CAD build for the part. Positions are in the model's coordinates, mm. A direction names the side the tool comes from. Round coordinates to 2 decimals unless told otherwise and drop trailing zeros. Order: outer loops, then holes, each group sorted by start corner. A loop starts at its lowest first (then second) coordinate and runs counter-clockwise, first axis right, second up. Notation, with made-up numbers: M -1,-13 L 37,-13 A22 ccw 37,-5 Z; hole C 51,86 d7. An arc over 180 degrees is marked long. Answer as a JSON object with one key per item and string values.
```python
from build123d import *

# Parameters (mm, degrees)
EXTRUDE_1_DEPTH     = 5
FILLET_1_R          = 2.5
EXTRUDE_2_DEPTH     = 8
FILLET_3_R          = 2.5
SKETCH_5_W          = 1.467751534
SKETCH_5_H          = 4.178210798
SKETCH_5_W_2        = 1.389566385
CUT_EXTRUDE_1_DEPTH = 20
EXTRUDE_3_DEPTH     = 38
SKETCH_7_W          = 2.4
SKETCH_7_H          = 1.7
CUT_EXTRUDE_2_DEPTH = 38


with BuildPart() as part:
    # 草图1 → 凸台-拉伸1 (new body)
    with BuildSketch(Plane.XY):
        Polygon((0, 0), (0, 28), (4, 28), (7.380946094, 20.749537704), (11.912485029, 22.862629012), (7.185351304, 33), (-5, 33), (-5, -5), (8, -5), (8, 0), align=None)
    extrude(amount=EXTRUDE_1_DEPTH)

    # 圆角1
    fillet_1_edges = [part.edges().sort_by_distance(p)[0] for p in [
        (9.646715562, 21.806083358, 0),
        (7.185351304, 33, 2.5),
        (11.912485029, 22.862629012, 2.5),
        (7.380946094, 20.749537704, 2.5),
        (9.646715562, 21.806083358, 5),
    ]]
    fillet(fillet_1_edges, radius=FILLET_1_R - 0.0001)  # a hair under: the kernel refuses the full size

    # 草图3 → 凸台-拉伸2 (add)
    with BuildSketch(Plane(origin=(0, 0, 0), x_dir=(0, 0, -1), z_dir=(1, 0, 0))):
        with BuildLine():
            Line((-5, 0), (0, 0))
            ThreePointArc((0, 0), (-2.5, 2.5), (-5, 0))
        make_face()
    extrude(amount=EXTRUDE_2_DEPTH)

    # 圆角3
    fillet_3_edges = [part.edges().sort_by_distance(p)[0] for p in [
        (8, -2.5, 0),
        (8, -5, 2.5),
        (8, -2.5, 5),
        (8, 2.5, 2.5),
    ]]
    fillet(fillet_3_edges, radius=FILLET_3_R - 0.0001)  # a hair under: the kernel refuses the full size

    # 草图4 → 旋转3 (revolve)
    with BuildSketch(Plane(origin=(4.4, 0, 0), x_dir=(0, 0, -1), z_dir=(1, 0, 0))):
        with BuildLine():
            Line((-5.5, 0), (0.5, 0))
            ThreePointArc((0.5, 0), (-2.5, 3), (-5.5, 0))
        make_face()
    revolve(axis=Axis((4.4, 0, 2.5), (0, 0, -1)))

    # 草图5 → 切除-拉伸1 (cut)
    with BuildSketch(Plane.ZY.offset(5)):
        with Locations((-0.733875767, -0.010051234)):
            Rectangle(SKETCH_5_W, SKETCH_5_H)
        with Locations((5.694783193, -0.010051234)):
            Rectangle(SKETCH_5_W_2, SKETCH_5_H)
    extrude(amount=-CUT_EXTRUDE_1_DEPTH, mode=Mode.SUBTRACT)

    # 草图6 → 凸台-拉伸3 (add)
    with BuildSketch(Plane.XZ.offset(5)):
        Polygon((-5, 2.5), (-5, 3.5), (-7, 3.5), (-7, 5), (-9, 5), (-11.5, 2.5), (-9, 0), (-7, 0), (-7, 1.5), (-5, 1.5), align=None)
    extrude(amount=-EXTRUDE_3_DEPTH)

    # 草图7 → 切除-拉伸2 (cut)
    with BuildSketch(Plane.XZ.offset(5)):
        with Locations((-6, 4.15)):
            Rectangle(SKETCH_7_W, SKETCH_7_H)
        with Locations((-6, 0.85)):
            Rectangle(SKETCH_7_W, SKETCH_7_H)
    extrude(amount=-CUT_EXTRUDE_2_DEPTH, mode=Mode.SUBTRACT)


solid = part.part
```
Item 1: Drop flat-ended pins along their axis: pin 1 Ø1.9 at (y, z) = (9.5, 4) entering from -X; pin 2 Ø0.8 at (y, z) = (5.5, 4.5) entering from +X; pin 3 Ø1.4 at (y, z) = (9, 0.5) entering from -X. Give the stop position or say it passes through.
Worked answers:
{"pin 1": "stops at x = -10.95", "pin 2": "stops at x = 0", "pin 3": "stops at x = -10.2"}
Item 2: 3-axis set-ups, long thin cutter, end or side, ignore diameter. For faces 1 (the flat face through (5.146, 25.543, 2.465)), 2 (the flat face through (-7.2, 14, 4)), 3 (the cylindrical face through (7.248, -1.979, 4.287)): which of +Z, -Z, +X, -X, +Y, -Y reach the whole face in a straight line?
Worked answers:
{"face 1": "+Z, -Z", "face 2": "+Z, +Y, -Y", "face 3": "+Z, +X, -Y"}
Item 3: Saw through at B-B on y = 27.5. List the corners of the cut face in (x, z).
Worked answers:
{"outline": "M -11.5,2.5 L -9,0 L -7.2,0 L -7.2,1.7 L -4.8,1.7 L -4.8,0 L 0,0 L 0,5 L -4.8,5 L -4.8,3.3 L -7.2,3.3 L -7.2,5 L -9,5 Z; M 4.23,0 L 9.75,0 L 9.75,5 L 4.23,5 Z"}
Item 4: Wall check: line 1 along X through (y, z) = (26.5, 0.7); line 2 along X through (y, z) = (23, 4.05); line 3 along Y through (x, z) = (1, 2.55). Give the ranges that are in metal, low to high. Write a range as [from, to].
Worked answers:
{"line 1": "x = [-9.7, -7.2], [-4.8, 0], [4.7, 10.22]", "line 2": "x = [-9.95, -7.2], [-4.8, 0], [6.33, 10.85]", "line 3": "y = [-5, 2.5], [28, 33]"}
Item 5: Saw through at C-C on y = 12. List the corners of the cut face in (x, z).
Worked answers:
{"outline": "M -11.5,2.5 L -9,0 L -7.2,0 L -7.2,1.7 L -4.8,1.7 L -4.8,0 L 0,0 L 0,5 L -4.8,5 L -4.8,3.3 L -7.2,3.3 L -7.2,5 L -9,5 Z"}
Item 6: Saw through at D-D on x = -5.5. List the corners of the cut face in (y, z), and give its area (3 significant figures).
Worked answers:
{"outline": "M -5,1.7 L 33,1.7 L 33,3.3 L -5,3.3 Z", "area": "60.8 mm2"}
Item 7: Two-plate mould, pull along Y, no slides. Class faces 4 (the cylindrical face through (1.4, 2.5, 2.4)), 5 (the flat face through (-1, 14, 5)), 6 (the flat face through (-1, 33, 2)), 7 (the cylindrical face through (9.237, 22.767, 4.532)): released by +Y, released by -Y, zero draft, split by the parting line, or undercut.
Worked answers:
{"face 4": "undercut", "face 5": "zero draft", "face 6": "released by +Y", "face 7": "released by -Y"}
Item 8: Saw through at A-A on x = 1.25. List the corners of the cut face in (y, z), and give its area (3 significant figures).
Worked answers:
{"outline": "M -5,0 L 0,0 A2.5 ccw 0,5 L -5,5 Z; M 28,0 L 33,0 L 33,5 L 28,5 Z", "area": "59.8 mm2"}
